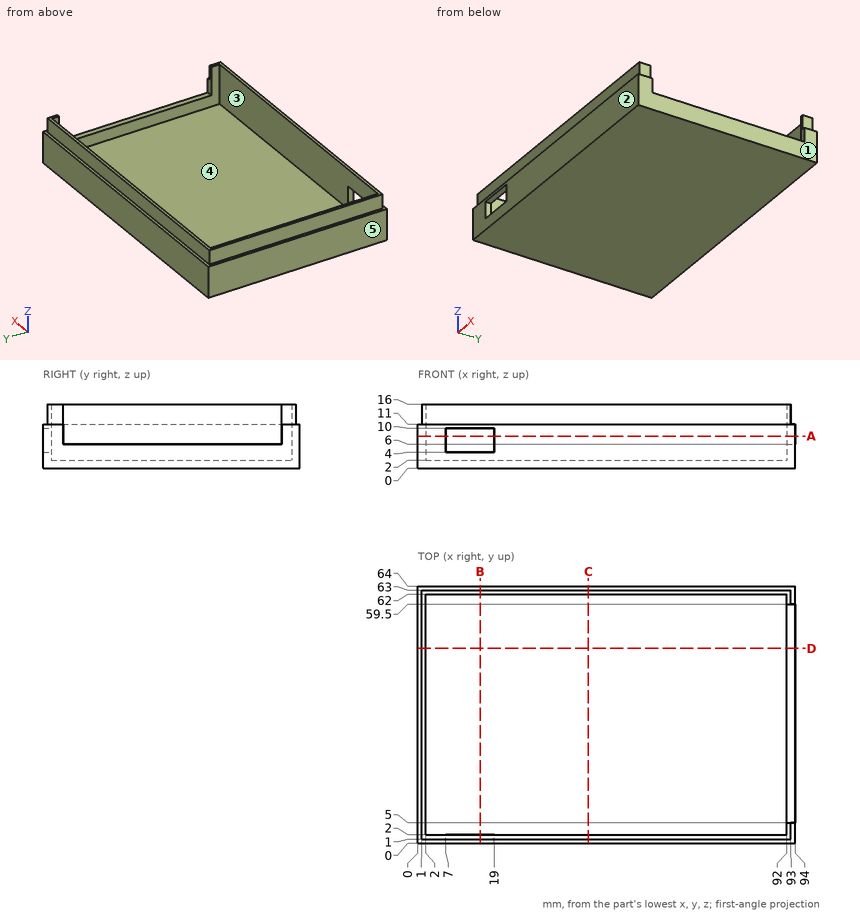
Design review of the part shown in the three views and the two pictorial views. Dimensions are in mm from the part's minimum x, y and z. A direction names the side the tool comes from. Round coordinates to 2 decimals unless told otherwise and drop trailing zeros. Loops run counter-clockwise (first coordinate to the right, second up) from the corner with the lowest first, then second, coordinate; pieces in that order, holes last. Notation, with made-up numbers: M 12.25,57 L 53.25,57 A15 ccw 53.25,70 Z; hole C 60,75.25 d2. An arc over 180 degrees is marked long. Answer as a JSON object with one key per item and string values.
Item 1: We need section A-A, the plane z = 8. State the section outline as (x, y) points, and give its area (3 significant figures).
Check sheet entries:
{"outline": "M 0,0 L 7,0 L 7,2 L 2,2 L 2,62 L 92,62 L 92,59.5 L 94,59.5 L 94,64 L 0,64 Z; M 19,0 L 94,0 L 94,5 L 92,5 L 92,2 L 19,2 Z", "area": "483 mm2"}
Item 2: Tool access review of the marked faces 4 and 5: name each direction out of +Z, -Z, +X, -X, +Y, -Y from which nothing blocks a thin tool from reaching the whole face with its end or side.
Check sheet entries:
{"face 4": "+Z", "face 5": "+Z, -Z, -X, +Y, -Y"}
Item 3: For line 1 along X through (y, z) = (16, 3); line 2 along Y through (x, z) = (27, 8.5); line 3 along Y through (x, z) = (31.5, 13.5), list the stretches that pass through material, from the lowest coordinate up.
Check sheet entries:
{"line 1": "0 to 2, 92 to 94", "line 2": "0 to 2, 62 to 64", "line 3": "1 to 2, 62 to 63"}
Item 4: We need section C-C, the plane x = 42.5. State the section outline as (y, z) points.
Check sheet entries:
{"outline": "M 0,0 L 64,0 L 64,11 L 63,11 L 63,16 L 62,16 L 62,2 L 2,2 L 2,16 L 1,16 L 1,11 L 0,11 Z"}
Item 5: We need section B-B, the plane x = 15.5. State the section outline as (y, z) points.
Check sheet entries:
{"outline": "M 0,0 L 64,0 L 64,11 L 63,11 L 63,16 L 62,16 L 62,2 L 2,2 L 2,4 L 0,4 Z; M 0,10 L 2,10 L 2,16 L 1,16 L 1,11 L 0,11 Z"}
Item 6: The part is to be moulded in two halves that separate along X. For the marked faces 1, 2 and 3, say which applies: +X half, -X half, draft (parallel to the pull), parting line (faces both ways), or undercut.
Check sheet entries:
{"face 1": "+X half", "face 2": "draft", "face 3": "undercut"}
Item 7: Clearance check with flat-ended pins moving along their axes: P1, Ø3, axis at x = 33, z = 3.5, coming from the -Y side; P2, Ø3, axis at y = 10, z = 13, coming from the -X side; P3, Ø1.6, axis at x = 93, y = 24, coming from the +Z side; P4, Ø2, axis at x = 81.5, y = 24.5, coming from the +Z side. State where each tip first meets the part, or that it passes through.
Check sheet entries:
{"P1": "y = 0", "P2": "x = 1", "P3": "z = 6", "P4": "z = 2"}
Item 8: We need section D-D, the plane y = 48.5. State the section outline as (x, z) points, and give its area (3 significant figures).
Check sheet entries:
{"outline": "M 0,0 L 94,0 L 94,6 L 92,6 L 92,2 L 2,2 L 2,16 L 1,16 L 1,11 L 0,11 Z", "area": "219 mm2"}
